```python
from build123d import *

# Parameters (mm, degrees)
IZIM1_W                          = 150
IZIM1_H                          = 70
Y_KSEKLIK_EKSTR_ZYON1_REACH      = 371.188
Y_KSEKLIK_EKSTR_ZYON1_END_RADIUS = 150
IZIM2_W                          = 79.999999942
IZIM2_H                          = 40
DELIK1_D                         = 260
F_6_8_6_8_AP_DELIK1_D            = 6.8
F_6_8_6_8_AP_DELIK1_DEPTH        = 40
IZIM10_R                         = 150
IZIM10_R_2                       = 130
KES_EKSTR_ZYON2_DEPTH            = 70
KES_EKSTR_ZYON3_START            = -20
KES_EKSTR_ZYON3_DEPTH            = 20


with BuildPart() as part:
    # Çizim1 → Döndür1 (revolve)
    with BuildSketch(Plane.XY, mode=Mode.PRIVATE) as d_nd_r1_sk:
        with Locations((75, 35)):
            Rectangle(IZIM1_W, IZIM1_H)
    revolve(d_nd_r1_sk.sketch.rotate(Axis((0, 70, 0), (0, -1, 0)), 270), axis=Axis((0, 70, 0), (0, -1, 0)))

    # Yükseklik-Ekstrüzyon1: up to this cylinder (the profile starts outside it)
    y_kseklik_ekstr_zyon1_end = Plane(origin=(0, 20, 0), z_dir=(0, -1, 0)) * Cylinder(Y_KSEKLIK_EKSTR_ZYON1_END_RADIUS, 1043.376, mode=Mode.PRIVATE)
    # Çizim2 → Yükseklik-Ekstrüzyon1 (add, up to the surface)
    with BuildSketch(Plane.XY.offset(180), mode=Mode.PRIVATE) as y_kseklik_ekstr_zyon1_sk1:
        with Locations((1e-08, 20)):
            Rectangle(IZIM2_W, IZIM2_H)
    y_kseklik_ekstr_zyon1_tool1 = extrude(y_kseklik_ekstr_zyon1_sk1.sketch, amount=-Y_KSEKLIK_EKSTR_ZYON1_REACH, mode=Mode.PRIVATE) - y_kseklik_ekstr_zyon1_end
    add(y_kseklik_ekstr_zyon1_tool1.solids().sort_by_distance((0, 20, 180))[0])

    # Delik1 (through all)
    with Locations(Plane(origin=(0, 70, 0), x_dir=(1, 0, 0), z_dir=(0, 1, 0))):
        with Locations((0, 0)):
            Hole(DELIK1_D / 2)

    # Ø6.8 (6.8) Çap Delik1
    with Locations(Plane(origin=(0, 40, 0), x_dir=(1, 0, 0), z_dir=(0, 1, 0))):
        with Locations((0, -162.284161474), (0, 162.284161474)):
            Hole(F_6_8_6_8_AP_DELIK1_D / 2, depth=F_6_8_6_8_AP_DELIK1_DEPTH)

    # Çizim10 → Kes-Ekstrüzyon2 (cut)
    with BuildSketch(Plane(origin=(0, 70, 0), x_dir=(1, 0, 0), z_dir=(0, 1, 0))):
        Circle(IZIM10_R)
        Circle(IZIM10_R_2, mode=Mode.SUBTRACT)
    extrude(amount=-KES_EKSTR_ZYON2_DEPTH, mode=Mode.SUBTRACT)

    # Çizim11 → Kes-Ekstrüzyon3 (cut)
    with BuildSketch(Plane.XZ.offset(KES_EKSTR_ZYON3_START)):
        with BuildLine():
            Line((39.999999981, 144.568322953), (39.999999981, 180))
            Line((39.999999981, 180), (-39.999999961, 180))
            Line((-39.999999961, 180), (-39.999999961, 144.568322959))
            ThreePointArc((-39.999999961, 144.568322959), (1e-08, 150), (39.999999981, 144.568322953))
        make_face()
    extrude(amount=KES_EKSTR_ZYON3_DEPTH, mode=Mode.SUBTRACT)


solid = part.part
```
Check sheet for the modelled part. Datum: model origin and axes. Units: mm. Coordinates: 2 decimals unless noted, no trailing zeros. Loops run counter-clockwise (first coordinate to the right, second up) from the corner with the lowest first, then second, coordinate; pieces in that order, holes last.
1) Sectioned sample at D-D (x = -29). Record the boundary of the cut face in (y, z).
2) Release check for a two-part mould opening along X. For faces 1 (the face through (-0.6, 30.1, 150)), 2 (the face through (-1, 40, 166)), 3 (the face through (-40, 30, 163)) record: released by +X, released by -X, zero draft, split by the parting line, or undercut.
3) Sectioned sample at A-A (x = 0). Record the boundary of the cut face in (y, z).
4) Gauge pin test, flat ends, axial feed: pin 1 (2 mm diameter, centred on x = 23, y = 24.5, fed in from -Z); pin 2 (2 mm diameter, centred on x = 26.5, y = 26, fed in from -Z); pin 3 (1.5 mm diameter, centred on x = 22, y = 29, fed in from -Z). Record the tip position at first contact, or that the pin passes through.
5) Sectioned sample at B-B (z = 164.5). Record the boundary of the cut face in (x, y), and give its area (3 significant figures).
6) Sectioned sample at C-C (y = 28.75). Record the boundary of the cut face in (x, z).
7) Material ranges on probe 1 along Z at (x, y) = (0, 31); probe 2 along X at (y, z) = (31, 160.5); probe 3 along Z at (x, y) = (-1.5, 23.25), recorded low to high.
Check sheet entries:
1. outline: (20, 147.17) - (40, 147.17) - (40, 180) - (20, 180) - close
2. face 1: undercut
2. face 2: zero draft
2. face 3: released by -X
3. outline: (20, 150) - (40, 150) - (40, 158.88) - (20, 158.88) - close; (20, 165.68) - (40, 165.68) - (40, 180) - (20, 180) - close
4. pin 1: stops at z = 148.07
4. pin 2: stops at z = 147.46
4. pin 3: stops at z = 148.26
5. outline: (-40, 20) - (-2.58, 20) - (-2.58, 40) - (-40, 40) - close; (2.58, 20) - (40, 20) - (40, 40) - (2.58, 40) - close
5. area: 1,500 mm2
6. outline: (-40, 144.57) arc R150 cw to (40, 144.57) - (40, 180) - (-40, 180) - close; hole circle Ø6.8 at (0, 162.28)
7. probe 1: z = 150 to 158.88, 165.68 to 180
7. probe 2: x = -40 to -2.89, 2.89 to 40
7. probe 3: z = 149.99 to 159.23, 165.34 to 180
